```python
from build123d import *

# Parameters (mm, degrees)
BOSS_EXTRUDE1_DEPTH = 53.34
SKETCH4_W           = 61.072672184
SKETCH4_H           = 27.686
CUT_EXTRUDE3_DEPTH  = 29.259495037
SKETCH5_OUTSIDE_W   = 57.352
SKETCH5_OUTSIDE_H   = 152.814
CUT_EXTRUDE5_DEPTH  = 54.34
SKETCH6_R           = 2.413
CUT_EXTRUDE6_DEPTH  = 54.34


with BuildPart() as part:
    # Sketch1 → Boss-Extrude1 (new body)
    with BuildSketch(Plane(origin=(0, 0, 0), x_dir=(1, 0, 0), z_dir=(0, 1, 0))):
        with BuildLine():
            Line((-13.944778991, -0.365156889), (-11.616850564, -89.265156889))
            ThreePointArc((-11.616850564, -89.265156889), (0, -109.412099434), (11.616850564, -89.265156889))
            Line((11.616850564, -89.265156889), (13.944778991, -0.365156889))
            ThreePointArc((13.944778991, -0.365156889), (0, 13.949559157), (-13.944778991, -0.365156889))
        make_face()
    extrude(amount=BOSS_EXTRUDE1_DEPTH)

    # Sketch4 → Cut-Extrude3 (cut, through all)
    with BuildSketch(Plane(origin=(13.944778991, 0, 0.365156889), x_dir=(0.026176948, 0, -0.999657325), z_dir=(0.999657325, 0, 0.026176948))):
        with Locations((0, 26.67)):
            Rectangle(SKETCH4_W, SKETCH4_H)
    extrude(amount=-CUT_EXTRUDE3_DEPTH, mode=Mode.SUBTRACT)

    # Sketch5 outside → Cut-Extrude5 (cut, through all)
    with BuildSketch(Plane(origin=(0, 53.34, 0), x_dir=(1, 0, 0), z_dir=(0, 1, 0))):
        with Locations((0, -47.731)):
            Rectangle(SKETCH5_OUTSIDE_W, SKETCH5_OUTSIDE_H)
        with BuildLine():
            Line((-13.944778991, -0.365156889), (-11.616850564, -89.265156889))
            ThreePointArc((-11.616850564, -89.265156889), (0, -109.412099434), (11.616850564, -89.265156889))
            Line((11.616850564, -89.265156889), (13.944778991, -0.365156889))
            ThreePointArc((13.944778991, -0.365156889), (0, 13.949559157), (-13.944778991, -0.365156889))
        make_face(mode=Mode.SUBTRACT)
        with BuildLine():
            Line((7.403977553, -7.568443783), (5.213735587, -91.210409969))
            ThreePointArc((5.213735587, -91.210409969), (0, -105.33899845), (-5.213735587, -91.210409969))
            Line((-5.213735587, -91.210409969), (-7.403977553, -7.568443783))
            Line((-7.403977553, -7.568443783), (7.403977553, -7.568443783))
        make_face()
    extrude(amount=-CUT_EXTRUDE5_DEPTH, mode=Mode.SUBTRACT)

    # Sketch6 → Cut-Extrude6 (cut, through all)
    with BuildSketch(Plane(origin=(0, 53.34, 0), x_dir=(1, 0, 0), z_dir=(0, 1, 0))):
        with Locations((0, 4.57874024)):
            Circle(SKETCH6_R)
    extrude(amount=-CUT_EXTRUDE6_DEPTH, mode=Mode.SUBTRACT)


solid = part.part
```
The model under review builds one solid part; all positions refer to its coordinate system, in mm. A direction names the side the tool comes from. Round coordinates to 2 decimals unless told otherwise and drop trailing zeros. Loops run counter-clockwise (first coordinate to the right, second up) from the corner with the lowest first, then second, coordinate; pieces in that order, holes last. Notation, with made-up numbers: M 35,66 L 48,66 A33 ccw 48,95 Z; hole C 21,31.5 d5. An arc over 180 degrees is marked long. Answer as a JSON object with one key per item and string values.
(1) Clearance check with flat-ended pins moving along their axes: P1, Ø6.5, axis at x = -0.5, y = 8, coming from the +Z side; P2, Ø1, axis at x = 8.5, y = 16, coming from the +Z side; P3, Ø6, axis at x = 5, y = 9.5, coming from the -Z side; P4, Ø1.5, axis at y = 23.5, z = 77.5, coming from the -X side. State where each tip first meets the part, or that it passes through.
Resolved:
{"P1": "z = 109.41", "P2": "z = 106.77", "P3": "z = -13.81", "P4": "x = -11.94"}
(2) Take a section at B-B on y = 34. Give the boundary of the cut face in (x, z), and give its area (3 significant figures).
Resolved:
{"outline": "M -13.16,30.2 L -6.81,30.37 L -5.21,91.21 A8.03 cw long 5.21,91.21 L 6.8,30.72 L 13.15,30.89 L 11.62,89.27 A13.42 ccw long -11.62,89.27 Z", "area": "993 mm²"}
(3) Take a section at D-D on x = -9.5. Give the boundary of the cut face in (y, z), and give its area (3 significant figures).
Resolved:
{"outline": "M 0,-10.21 L 12.83,-10.21 L 12.83,30.3 L 40.51,30.3 L 40.51,-10.21 L 53.34,-10.21 L 53.34,105.47 L 0,105.47 Z", "area": "5,050 mm²"}
(4) Take a section at C-C on z = 77.5. Give the boundary of the cut face in (x, y), and give its area (3 significant figures).
Resolved:
{"outline": "M -11.92,0 L -5.57,0 L -5.57,53.34 L -11.92,53.34 Z; M 5.57,0 L 11.92,0 L 11.92,53.34 L 5.57,53.34 Z", "area": "678 mm²"}
(5) To check wall thickness, follow line 1 along Y through (x, z) = (-3, -3); line 2 along X through (y, z) = (17.5, 79); line 3 along X through (y, z) = (44.5, 12). State the ranges of each line that lie inside material, in increasing order.
Resolved:
{"line 1": "0 to 12.83, 40.51 to 53.34", "line 2": "-11.89 to -5.53, 5.53 to 11.89", "line 3": "-13.64 to -7.29, 7.29 to 13.64"}
(6) Tool access review of faces 3 (the flat face through (-9, 0, 33)), 4 (the flat face through (0, 47, 7.568)): name each direction out of +Z, -Z, +X, -X, +Y, -Y from which nothing blocks a thin tool from reaching the whole face with its end or side.
Resolved:
{"face 3": "+Z, -Z, +X, -X, -Y", "face 4": "+Y, -Y"}
(7) Take a section at A-A on x = 0. Give the boundary of the cut face in (y, z).
Resolved:
{"outline": "M 0,-13.95 L 12.83,-13.95 L 12.83,-6.99 L 0,-6.99 Z; M 0,-2.17 L 12.83,-2.17 L 12.83,7.57 L 0,7.57 Z; M 0,105.34 L 53.34,105.34 L 53.34,109.41 L 0,109.41 Z; M 40.51,-13.95 L 53.34,-13.95 L 53.34,-6.99 L 40.51,-6.99 Z; M 40.51,-2.17 L 53.34,-2.17 L 53.34,7.57 L 40.51,7.57 Z"}
(8) Draft analysis for pull direction Z (two halves, no side actions). For faces 1 (the cylindrical face through (-0.394, 26.297, 109.406)), 2 (the flat face through (0, 12.827, 4)), state which applies: released by +Z, released by -Z, zero draft, split by the parting line, or undercut.
Resolved:
{"face 1": "undercut", "face 2": "zero draft"}
